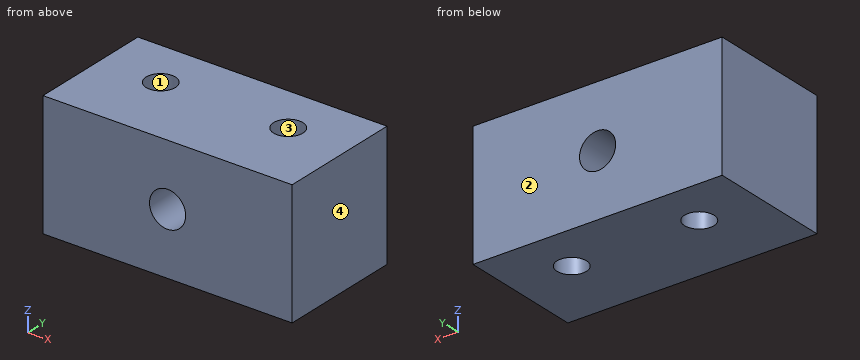
```python
from build123d import *

# Parameters (mm, degrees)
SKETCH1_W           = 25.4
SKETCH1_H           = 12.7
BOSS_EXTRUDE1_DEPTH = 12.7
SKETCH2_R           = 1.5
CUT_EXTRUDE1_DEPTH  = 32.108519733
SKETCH3_R           = 1.8415
CUT_EXTRUDE2_DEPTH  = 32.108519733


with BuildPart() as part:
    # Sketch1 → Boss-Extrude1 (new body)
    with BuildSketch(Plane(origin=(0, 0, 0), x_dir=(1, 0, 0), z_dir=(0, 1, 0))):
        with Locations((12.7, 6.35)):
            Rectangle(SKETCH1_W, SKETCH1_H)
    extrude(amount=BOSS_EXTRUDE1_DEPTH)

    # Sketch2 → Cut-Extrude1 (cut, through all)
    with BuildSketch(Plane.XY):
        with Locations((6.2, 7.62)):
            Circle(SKETCH2_R)
        with Locations(Location((19.2, 7.62, 0), (0, 0, 180))):
            Circle(SKETCH2_R)
    extrude(amount=-CUT_EXTRUDE1_DEPTH, mode=Mode.SUBTRACT)

    # Sketch3 → Cut-Extrude2 (cut, through all)
    with BuildSketch(Plane(origin=(0, 12.7, 0), x_dir=(1, 0, 0), z_dir=(0, 1, 0))):
        with Locations(Location((12.7, 6.35, 0), (0, 0, 270))):
            Circle(SKETCH3_R)
    extrude(amount=-CUT_EXTRUDE2_DEPTH, mode=Mode.SUBTRACT)


solid = part.part
```
CAD build for the part. Positions are in the model's coordinates, mm. Face numbers are marked on the shaded views. Round coordinates to 2 decimals unless told otherwise and drop trailing zeros. Order: outer loops, then holes, each group sorted by start corner. A loop starts at its lowest first (then second) coordinate and runs counter-clockwise, first axis right, second up.
Item 1: Probe line 1 along Y through (x, z) = (19.2, -6.5); line 2 along X through (y, z) = (7.25, -5.75); line 3 along X through (y, z) = (4.25, -6.35). List the from-to ranges inside material, lowest first.
Item 2: Mould opens along Y. For the marked faces 1, 2, 3 and 4 say: pulls with the +Y half, pulls with the -Y half, needs draft (parallel to the pull), parting line crosses it, or undercut.
Item 3: Saw through at B-B on y = 7.62. Write the cut outline in (x, z), then the cut area to 3 significant figures.
Item 4: Saw through at A-A on z = -6.35. Write the cut outline in (x, y), then the cut area to 3 significant figures.
Item 5: Saw through at D-D on y = 11.5. Write the cut outline in (x, z), then the cut area to 3 significant figures.
Item 6: Saw through at C-C on x = 6.2. Write the cut outline in (y, z), then the cut area to 3 significant figures.
Reported:
1. line 1: y = 0 to 6.12, 9.12 to 12.7
1. line 2: x = 0 to 4.75, 7.65 to 10.96, 14.44 to 17.75, 20.65 to 25.4
1. line 3: x = 0 to 10.86, 14.54 to 25.4
2. face 1: undercut
2. face 2: pulls with the +Y half
2. face 3: undercut
2. face 4: needs draft
3. outline: (0, -12.7) - (4.7, -12.7) - (4.7, 0) - (0, 0) - close; (7.7, -12.7) - (17.7, -12.7) - (17.7, 0) - (7.7, 0) - close; (20.7, -12.7) - (25.4, -12.7) - (25.4, 0) - (20.7, 0) - close; hole circle Ø3.68 at (12.7, -6.35)
3. area: 236 mm2
4. outline: (0, 0) - (10.86, 0) - (10.86, 12.7) - (0, 12.7) - close; (14.54, 0) - (25.4, 0) - (25.4, 12.7) - (14.54, 12.7) - close; hole circle Ø3 at (6.2, 7.62); hole circle Ø3 at (19.2, 7.62)
4. area: 262 mm2
5. outline: (0, -12.7) - (25.4, -12.7) - (25.4, 0) - (0, 0) - close; hole circle Ø3.68 at (12.7, -6.35)
5. area: 312 mm2
6. outline: (0, -12.7) - (6.12, -12.7) - (6.12, 0) - (0, 0) - close; (9.12, -12.7) - (12.7, -12.7) - (12.7, 0) - (9.12, 0) - close
6. area: 123 mm2
